Verification items for the finished model (mm, model axes). Face numbers are marked on the shaded views. A direction names the side the tool comes from. Round coordinates to 2 decimals unless told otherwise and drop trailing zeros. Loops run counter-clockwise (first coordinate to the right, second up) from the corner with the lowest first, then second, coordinate; pieces in that order, holes last. Notation, with made-up numbers: (-5, 60) -> (35, 60) arc R5 ccw to (35, 68) -> close; hole circle Ø11 at (-24, 65.5). An arc over 180 degrees is marked (long way). Use a Markdown table: item, result. Add a question column.
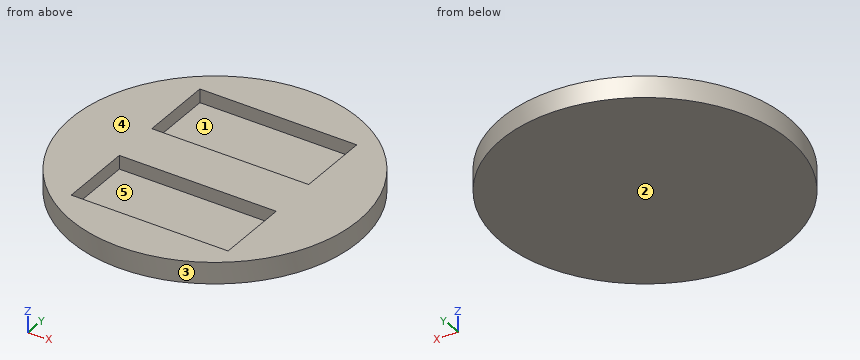
```python
from build123d import *

# Parameters (mm, degrees)
F0_R     = 27.5
F1_DEPTH = 4.1
F2_W     = 30
F2_H     = 14
F3_DEPTH = 2.6
F4_W     = 30
F4_H     = 14
F5_DEPTH = 2.6


with BuildPart() as f1:
    # F0 (on Top) → F1 (new body)
    with BuildSketch(Plane.XY):
        Circle(F0_R)
    extrude(amount=F1_DEPTH)

    # F2 (on face) → F3 (cut)
    with BuildSketch(Plane.XY.offset(4.1)):
        with Locations((0, 11.4413)):
            Rectangle(F2_W, F2_H)
    extrude(amount=-F3_DEPTH, mode=Mode.SUBTRACT)

    # F4 (on face) → F5 (cut)
    with BuildSketch(Plane.XY.offset(4.1)):
        with Locations((0, -12)):
            Rectangle(F4_W, F4_H)
    extrude(amount=-F5_DEPTH, mode=Mode.SUBTRACT)


solid = f1.part
```
1) Access from +Z, -Z, +X, -X, +Y, -Y to the whole of each face (thin tool, end or side, straight path). Record for the marked faces 1 and 2.
2) Release check for a two-part mould opening along Y. For the marked faces 3, 4 and 5 record: released by +Y, released by -Y, zero draft, split by the parting line, or undercut.
3) Sectioned sample at D-D on x = 12.5. Enter the section's corners in (y, z), then the cut area to 3 significant figures.
4) Go/stop test with flat-tipped pins: pin 1 (1.3 mm diameter, centred on y = 12.5, z = 2.5, fed in from -X); pin 2 (2 mm diameter, centred on x = -3, z = 2.5, fed in from +Y); pin 3 (1.5 mm diameter, centred on y = -5.5, z = 1.5, fed in from -X). Record where each tip stops, or that it passes through.
5) Thickness scan on line 1 (Y direction, x = 6, z = 1.65); line 2 (Z direction, x = -10, y = -13.5); line 3 (X direction, y = -16.5, z = 3.4). Record the ranges inside material, lowest first.
6) Sectioned sample at A-A on x = 0. Enter the section's corners in (y, z).
7) Sectioned sample at C-C on y = 7. Enter the section's corners in (x, z), then the cut area to 3 significant figures.
8) Sectioned sample at B-B on z = 3.35. Enter the section's corners in (x, y), then the cut area to 3 significant figures.
Geometry results:
| question | item | result |
|---|---|---|
| 1 | face 1 | +Z |
| 1 | face 2 | -Z, +X, -X, +Y, -Y |
| 2 | face 3 | split by the parting line |
| 2 | face 4 | zero draft |
| 2 | face 5 | undercut |
| 3 | outline | (-24.49, 0) -> (24.49, 0) -> (24.49, 4.1) -> (18.44, 4.1) -> (18.44, 1.5) -> (4.44, 1.5) -> (4.44, 4.1) -> (-5, 4.1) -> (-5, 1.5) -> (-19, 1.5) -> (-19, 4.1) -> (-24.49, 4.1) -> close |
| 3 | area | 128 mm^2 |
| 4 | pin 1 | x = -24.82 |
| 4 | pin 2 | y = 27.43 |
| 4 | pin 3 | x = -27.09 |
| 5 | line 1 | -26.84 to -19, -5 to 4.44, 18.44 to 26.84 |
| 5 | line 2 | 0 to 1.5 |
| 5 | line 3 | -22 to -15, 15 to 22 |
| 6 | outline | (-27.5, 0) -> (27.5, 0) -> (27.5, 4.1) -> (18.44, 4.1) -> (18.44, 1.5) -> (4.44, 1.5) -> (4.44, 4.1) -> (-5, 4.1) -> (-5, 1.5) -> (-19, 1.5) -> (-19, 4.1) -> (-27.5, 4.1) -> close |
| 7 | outline | (-26.59, 0) -> (26.59, 0) -> (26.59, 4.1) -> (15, 4.1) -> (15, 1.5) -> (-15, 1.5) -> (-15, 4.1) -> (-26.59, 4.1) -> close |
| 7 | area | 140 mm^2 |
| 8 | outline | circle Ø55 at (0, 0); hole (-15, -19) -> (15, -19) -> (15, -5) -> (-15, -5) -> close; hole (-15, 4.44) -> (15, 4.44) -> (15, 18.44) -> (-15, 18.44) -> close |
| 8 | area | 1,540 mm^2 |
